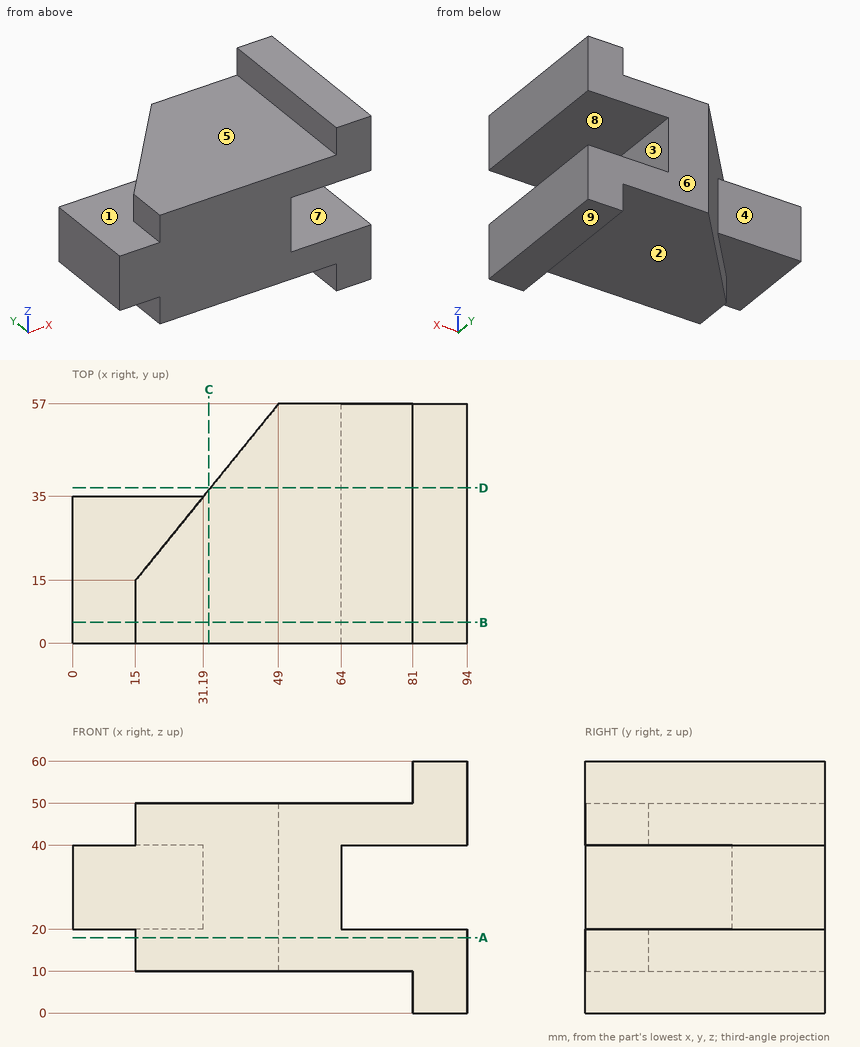
Geometry: see drawing. Coordinates: mm, zero at the bounding-box minimum. A direction names the side the tool comes from. Coordinates: 2 decimals unless noted, no trailing zeros. Loops run counter-clockwise (first coordinate to the right, second up) from the corner with the lowest first, then second, coordinate; pieces in that order, holes last. Notation, with made-up numbers: (28.25, 41.25) - (68.25, 41.25) arc R23 ccw to (68.25, 51.25) - close; hole circle Ø5 at (-34.75, 68). An arc over 180 degrees is marked (long way). Return JSON: item names as keys, results as strings.
Q1. Material intervals for line 1 along Z through (x, y) = (88.5, 19.5); line 2 along Z through (x, y) = (78, 20.5); line 3 along Z through (x, y) = (9.5, 31), sorted ascending.
Results:
{"line 1": "0 to 20, 40 to 60", "line 2": "10 to 20, 40 to 50", "line 3": "20 to 40"}
Q2. Section A-A, the plane z = 18. Return loops of the section in (x, y), plus the area to 3 significant figures.
Results:
{"outline": "(15, 0) - (94, 0) - (94, 57) - (49, 57) - (15, 15) - close", "area": "3,790 mm2"}
Q3. Mould query, pull axis Z, two halves, no side actions, for the marked faces 6, 7, 8 and 9. Classes: released by +Z, released by -Z, zero draft, split by the parting line, or undercut.
Results:
{"face 6": "zero draft", "face 7": "undercut", "face 8": "undercut", "face 9": "released by -Z"}
Q4. Section D-D, the plane y = 37. Return loops of the section in (x, z).
Results:
{"outline": "(32.81, 10) - (81, 10) - (81, 0) - (94, 0) - (94, 20) - (64, 20) - (64, 40) - (94, 40) - (94, 60) - (81, 60) - (81, 50) - (32.81, 50) - close"}
Q5. Section C-C, the plane x = 32.5. Return loops of the section in (y, z).
Results:
{"outline": "(0, 10) - (36.62, 10) - (36.62, 50) - (0, 50) - close"}
Q6. Contact query for flat-ended pins moving along their axis: P1, Ø6, axis at y = 17, z = 11, coming from the -X side; P2, Ø25, axis at x = 15, y = 26, coming from the -Z side; P3, Ø15, axis at x = 77, y = 40, coming from the -Z side; P4, Ø6, axis at x = 69.5, y = 36.5, coming from the +Z side. Output: stop coordinate, or through.
Results:
{"P1": "x = 15", "P2": "z = 10", "P3": "z = 0", "P4": "z = 50"}
Q7. Access query for the marked faces 1, 2, 3, 4 and 5. Directions: +Z, -Z, +X, -X, +Y, -Y. A direction counts if a zero-diameter tool reaches every point of the face in a straight line with its end or side. Return the directions, or none.
Results:
{"face 1": "+Z, -X, +Y", "face 2": "-Z, -X, +Y, -Y", "face 3": "+X, +Y, -Y", "face 4": "+Z, -Z, -X, +Y", "face 5": "+Z, -X, +Y, -Y"}
Q8. Section B-B, the plane y = 5. Return loops of the section in (x, z), plus the area to 3 significant figures.
Results:
{"outline": "(0, 20) - (15, 20) - (15, 10) - (81, 10) - (81, 0) - (94, 0) - (94, 20) - (64, 20) - (64, 40) - (94, 40) - (94, 60) - (81, 60) - (81, 50) - (15, 50) - (15, 40) - (0, 40) - close", "area": "3,120 mm2"}
